Read the model definition and answer for the solid it produces. Units are mm, in the model's axes. A direction names the side the tool comes from. Coordinates: 2 decimals unless noted, no trailing zeros. Write each loop counter-clockwise with the first axis right and the second up, starting at its lowest first coordinate (ties: lowest second). Pieces come first, ordered by that corner, then holes.
(1) Straight lines are drawn through the part: line 1 along Y through (x, z) = (10, 10); line 2 along X through (y, z) = (6.25, 0); line 3 along X through (y, z) = (5.35, 13.5). For each, find the intervals that lie inside material, in ascending order.
(2) The part is cut by section A-A, the plane z = 0. Determine the outline of the cut face in (x, y).
(3) The part is cut by section B-B, the plane x = 13. Determine the outline of the cut face in (y, z).
(4) Determine the mould class of faces 4 (the flat face through (-1, 6, -16)), 5 (the cylindrical face through (0.05, 5.49, 12.25)), 6 (the cylindrical face through (0.434, 1.298, -19.944)) for opening direction X: pulls with the +X half, pulls with the -X half, needs draft (parallel to the pull), parting line crosses it, or undercut.
(5) The part is cut by section C-C, the plane y = 0.5. Determine the outline of the cut face in (x, z).
(6) Which of the six approach directions +Z, -Z, +X, -X, +Y, -Y give full straight-line access (tool end or side, diameter ignored) to faces 1 (the flat face through (-1, 3, -11)), 2 (the flat face through (-1, 1, -16)), 3 (the flat face through (2, 3, -13))?
(7) Given pin 1 (0.6 mm diameter, centred on x = -1, y = 5.5, fed in from -Z); pin 2 (1 mm diameter, centred on y = 1.5, z = -12.5, fed in from -X); pin 3 (1 mm diameter, centred on x = 0.5, y = 3, fed in from +Z), each flat-ended and moving along its own axis, determine where each tip first touches the part or whether it passes through.
(8) The part is cut by section D-D, the plane x = 5. Determine the outline of the cut face in (y, z), and give its area (3 significant figures).
```python
from build123d import *

# Parameters (mm, degrees)
SKETCH1_R           = 1.25
BOSS_EXTRUDE1_DEPTH = 2
LPATTERN1_COUNT     = 2
LPATTERN1_PITCH     = 4.5
BOSS_EXTRUDE2_DEPTH = 2.5
SKETCH4_R           = 2
BOSS_EXTRUDE3_DEPTH = 8


with BuildPart() as part:
    # Sketch1 → Boss-Extrude1 (new body)
    with BuildSketch(Plane(origin=(0, 0, 0), x_dir=(1, 0, 0), z_dir=(0, 1, 0))):
        with BuildLine():
            Line((0, 11), (-2, 11))
            Line((-2, 11), (-2, 16))
            Line((-2, 16), (0, 16))
            ThreePointArc((0, 16), (16, 0), (0, -16))
            ThreePointArc((0, -16), (-2.5, -13.5), (0, -11))
            ThreePointArc((0, -11), (11, 0), (0, 11))
        make_face()
        with Locations(Location((0, -13.5, 0), (0, 0, 270))):
            Circle(SKETCH1_R, mode=Mode.SUBTRACT)
    extrude(amount=BOSS_EXTRUDE1_DEPTH)


with BuildPart() as lpattern1_1:
    # LPattern1: pattern copy
    add(part.part.moved(Location(Vector(0, 1, 0) * (1 * LPATTERN1_PITCH))))


with BuildPart() as part_1:
    add(part.part)

    add(lpattern1_1.part)  # Boss-Extrude2 merges LPattern1_1
    # Sketch3 → Boss-Extrude2 (add)
    with BuildSketch(Plane(origin=(0, 2, 0), x_dir=(1, 0, 0), z_dir=(0, 1, 0))):
        with BuildLine():
            Line((-2, 16), (-2, 11))
            Line((-2, 11), (0, 11))
            ThreePointArc((0, 11), (1.004193186, 10.954067557), (2, 10.816653826))
            Line((2, 10.816653826), (2, 15.874507866))
            ThreePointArc((2, 15.874507866), (1.001966601, 15.968596148), (0, 16))
            Line((0, 16), (-2, 16))
        make_face()
    extrude(amount=BOSS_EXTRUDE2_DEPTH)

    # Sketch4 → Boss-Extrude3 (add)
    with BuildSketch(Plane(origin=(0, 0, -16), x_dir=(-1, 0, 0), z_dir=(0, 0, -1))):
        with Locations((0, 3.25)):
            Circle(SKETCH4_R)
    extrude(amount=BOSS_EXTRUDE3_DEPTH)


solid = part_1.part
```
Computed:
1. line 1: y = 0 to 2, 4.5 to 6.5
1. line 2: x = 11 to 16
1. line 3: x = -2.5 to -1.25, 1.25 to 8.59
2. outline: (11, 0) - (16, 0) - (16, 2) - (11, 2) - close; (11, 4.5) - (16, 4.5) - (16, 6.5) - (11, 6.5) - close
3. outline: (0, -9.33) - (2, -9.33) - (2, 9.33) - (0, 9.33) - close; (4.5, -9.33) - (6.5, -9.33) - (6.5, 9.33) - (4.5, 9.33) - close
4. face 4: needs draft
4. face 5: undercut
4. face 6: parting line crosses it
5. outline: (-2, -16) - (0, -16) arc R16 ccw to (0, 16) arc R2.5 ccw to (0, 11) arc R11 cw to (0, -11) - (-2, -11) - close; hole circle Ø2.5 at (0, 13.5)
6. face 1: -X, +Y, -Y
6. face 2: -Z, -X, -Y
6. face 3: +Z, -Z, +X
7. pin 1: stops at z = -16
7. pin 2: stops at x = -2
7. pin 3: stops at z = -10.95
8. outline: (0, -15.2) - (2, -15.2) - (2, -9.8) - (0, -9.8) - close; (0, 9.8) - (2, 9.8) - (2, 15.2) - (0, 15.2) - close; (4.5, -15.2) - (6.5, -15.2) - (6.5, -9.8) - (4.5, -9.8) - close; (4.5, 9.8) - (6.5, 9.8) - (6.5, 15.2) - (4.5, 15.2) - close
8. area: 43.2 mm2
